The model under review builds one solid part; all positions refer to its coordinate system, in mm. A direction names the side the tool comes from. Give positions to 0.01 mm unless a question says otherwise; leave off trailing zeros. Order: outer loops, then holes, each group sorted by start corner. A loop starts at its lowest first (then second) coordinate and runs counter-clockwise, first axis right, second up. Notation, with made-up numbers: (47, 67.25) - (71, 67.25) arc R25 cw to (71, 96.25) - close; hole circle Ø1 at (72, -14.5). An arc over 180 degrees is marked (long way). Use CSV: the item, a comma, the result in double quotes. Start each with the question number.
1. For pin 1 (1 mm diameter, centred on y = 13.5, z = 8, fed in from -X); pin 2 (4 mm diameter, centred on x = 20, y = 22.5, fed in from +Z); pin 3 (5 mm diameter, centred on x = -1, y = 11, fed in from -Z); pin 4 (3 mm diameter, centred on x = -15, z = 14.5, fed in from -Y), all flat-tipped, find the tip position at first contact; note any pin that passes through.
2. Draft analysis for pull direction Z (two halves, no side actions). For faces 1 (the cylindrical face through (4.231, 42.919, 32.223)), 2 (the cylindrical face through (14.079, 3.944, 15.845)), 3 (the flat face through (13, 41, -14.195)), state which applies: released by +Z, released by -Z, zero draft, split by the parting line, or undercut.
3. Machinability: for faces 4 (the flat face through (0, 0, 0)), 5 (the flat face through (-15, 8, -15)), 6 (the flat face through (-13, 41, -14.195)), which of the approach directions +Z, -Z, +X, -X, +Y, -Y give a long, thin tool a straight path to every point of the face, cutting with its end or side? Answer none if there is none.
4. Take a section at A-A, the plane x = 0. State the section outline as (y, z) points, then the cut area to 3 significant figures.
5. Take a section at B-B, the plane z = 0. State the section outline as (x, y) points.
6. Take a section at C-C, the plane y = 49. State the section outline as (x, z) points, then the cut area to 3 significant figures.
7. To check wall thickness, follow line 1 (Z direction, x = -15, y = 3); line 2 (Y direction, x = -25.5, z = 15.5); line 3 (Y direction, x = 15.5, z = 15.5). State the ranges of each line that lie inside material, in increasing order. Write a range as [from, to].
8. Take a section at D-D, the plane y = 15.5. State the section outline as (x, z) points, then the cut area to 3 significant figures.
```python
from build123d import *

# Parameters (mm, degrees)
SKETCH3_R          = 1.25
CUT_EXTRUDE1_DEPTH = 8


with BuildPart() as part:
    # Sketch1 → Revolve1 (revolve)
    with BuildSketch(Plane.XY):
        Polygon((0, 0), (-23.5, 0), (-23.5, 2), (-25.5, 2), (-25.5, 23.4), (-32.5, 23.4), (-32.5, 61.9), (0, 61.9), align=None)
    revolve(axis=Axis((0, -426.088089194, 0), (0, 1, 0)))

    # Sketch2 → Cut-Revolve1 (revolve, cut)
    with BuildSketch(Plane(origin=(0, 41.5, 0), x_dir=(-1, 0, 0), z_dir=(0, -1, 0))):
        Polygon((-19.929871148, 32.5), (-19.85, 14.194997457), (-13.5, 14.194997457), (-13.5, 32.5), align=None)
    cut_revolve1 = revolve(axis=Axis((13.5, 41.5, 985.805002543), (0, 0, -1)), mode=Mode.SUBTRACT)

    # Mirror1: Cut-Revolve1 across plane
    add(cut_revolve1.mirror(Plane(origin=(0, 0, 0), x_dir=(0, 0, 1), z_dir=(1, 0, 0))), mode=Mode.SUBTRACT)

    # Sketch3 → Cut-Extrude1 (cut)
    with BuildSketch(Plane.XZ):
        with Locations((-15, 15)):
            Circle(SKETCH3_R)
        with Locations((-15, -15)):
            Circle(SKETCH3_R)
        with Locations((15, -15)):
            Circle(SKETCH3_R)
        with Locations((15, 15)):
            Circle(SKETCH3_R)
    extrude(amount=-CUT_EXTRUDE1_DEPTH, mode=Mode.SUBTRACT)


solid = part.part
```
Determined:
1,pin 1,"stops at x = -24.37"
1,pin 2,"stops at z = 26.92"
1,pin 3,"stops at z = -25.5"
1,pin 4,"stops at y = 0"
2,face 1,"split by the parting line"
2,face 2,"undercut"
2,face 3,"released by -Z"
3,face 4,"+Z, -Z, +X, -X, -Y"
3,face 5,"-Y"
3,face 6,"-Z"
4,outline,"(0, -23.5) - (2, -23.5) - (2, -25.5) - (23.4, -25.5) - (23.4, -32.5) - (61.9, -32.5) - (61.9, 32.5) - (23.4, 32.5) - (23.4, 25.5) - (2, 25.5) - (2, 23.5) - (0, 23.5) - close"
4,area,"3,690 mm²"
5,outline,"(-32.5, 23.4) - (-25.5, 23.4) - (-25.5, 2) - (-23.5, 2) - (-23.5, 0) - (23.5, 0) - (23.5, 2) - (25.5, 2) - (25.5, 23.4) - (32.5, 23.4) - (32.5, 61.9) - (-32.5, 61.9) - close"
6,outline,"circle Ø65 at (0, 0)"
6,area,"3,320 mm²"
7,line 1,"z = [-20.62, -16.25], [-13.75, 13.75], [16.25, 20.62]"
7,line 2,"y = [23.4, 61.9]"
7,line 3,"y = [8, 61.9]"
8,outline,"circle Ø51 at (0, 0)"
8,area,"2,040 mm²"
